Geometry check sheet. Reference: the model listing, model coordinates, mm. A direction names the side the tool comes from. Round coordinates to 2 decimals unless told otherwise and drop trailing zeros. Order: outer loops, then holes, each group sorted by start corner. A loop starts at its lowest first (then second) coordinate and runs counter-clockwise, first axis right, second up. Notation, with made-up numbers: (-5, 0) - (24, 0) arc R7 cw to (24, 10) - close; hole circle Ø2 at (53.5, 59.25). An arc over 180 degrees is marked (long way). Use a Markdown table: item, result. Add a question column.
(1) Access from +Z, -Z, +X, -X, +Y, -Y to the whole of each face (thin tool, end or side, straight path). Record for faces 4 (the face through (0, -22, 8)), 5 (the face through (12.5, -41, 4)).
(2) Gauge pin test, flat ends, axial feed: P1, Ø4, axis at y = -39.5, z = 6, coming from the -X side; P2, Ø2, axis at x = 10.5, z = 2, coming from the +Y side. Record the tip position at first contact, or that the pin passes through.
(3) Thickness scan on line 1 along Y through (x, z) = (0, 3.75); line 2 along Y through (x, z) = (0, 3.5); line 3 along X through (y, z) = (-49.5, 6). Record the ranges inside material, lowest first. Write a range as [from, to].
(4) Section check B-B on x = 0. Record the boundary of the cut face in (y, z), then the cut area to 3 significant figures.
(5) Section check C-C on y = -57.5. Record the boundary of the cut face in (x, z).
(6) Section check A-A on z = 4. Record the boundary of the cut face in (x, y).
(7) Mould release check, pull along Y, two halves, no side actions. Record for faces 1 (the face through (-14.985, 0.66, 3.944)), 2 (the face through (-12.5, -40, 4)), 3 (the face through (0, -65.612, 4)): released by +Y, released by -Y, zero draft, split by the parting line, or undercut.
(8) Section check D-D on x = 4.5. Record the boundary of the cut face in (y, z), then the cut area to 3 significant figures.
```python
from build123d import *

# Parameters (mm, degrees)
F0_R     = 15
F1_DEPTH = 8
F3_D     = 6


with BuildPart() as f1:
    # F0 (on Top) → F1 (new body)
    with BuildSketch(Plane.XY):
        with BuildLine():
            ThreePointArc((12.5, -15.612494996), (18.0277563773, -8.6602540378), (20, 0))
            ThreePointArc((20, 0), (-8.6602540378, 18.0277563773), (-12.5, -15.612494996))
            Line((-12.5, -15.612494996), (12.5, -15.612494996))
        make_face()
        Circle(F0_R, mode=Mode.SUBTRACT)
        with BuildLine():
            Line((12.5, -15.612494996), (-12.5, -15.612494996))
            ThreePointArc((-12.5, -15.612494996), (0, -20), (12.5, -15.612494996))
        make_face()
        with BuildLine():
            ThreePointArc((12.5, -15.612494996), (0, -20), (-12.5, -15.612494996))
            Line((-12.5, -15.612494996), (-12.5, -65.612494996))
            Line((-12.5, -65.612494996), (12.5, -65.612494996))
            Line((12.5, -65.612494996), (12.5, -15.612494996))
        make_face()
    extrude(amount=F1_DEPTH)

    # F3 (through all)
    with Locations(Plane.YZ.offset(12.5)):
        with Locations((-55.612494996, 4)):
            Hole(F3_D / 2)


solid = f1.part
```
Check sheet entries:
| question | item | result |
|---|---|---|
| 1 | face 4 | +Z, +X, -X, +Y, -Y |
| 1 | face 5 | +Z, -Z, +X, -Y |
| 2 | P1 | stops at x = -12.5 |
| 2 | P2 | stops at y = 17.6 |
| 3 | line 1 | y = [-65.61, -58.6], [-52.62, -15], [15, 20] |
| 3 | line 2 | y = [-65.61, -58.57], [-52.65, -15], [15, 20] |
| 3 | line 3 | x = [-12.5, 12.5] |
| 4 | outline | (-65.61, 0) - (-15, 0) - (-15, 8) - (-65.61, 8) - close; (15, 0) - (20, 0) - (20, 8) - (15, 8) - close; hole circle Ø6 at (-55.61, 4) |
| 4 | area | 417 mm2 |
| 5 | outline | (-12.5, 0) - (12.5, 0) - (12.5, 1.67) - (-12.5, 1.67) - close; (-12.5, 6.33) - (12.5, 6.33) - (12.5, 8) - (-12.5, 8) - close |
| 6 | outline | (-12.5, -65.61) - (12.5, -65.61) - (12.5, -58.61) - (-12.5, -58.61) - close; (-12.5, -52.61) - (12.5, -52.61) - (12.5, -15.61) arc R20 ccw (long way) to (-12.5, -15.61) - close; hole circle Ø30 at (0, 0) |
| 7 | face 1 | undercut |
| 7 | face 2 | zero draft |
| 7 | face 3 | released by -Y |
| 8 | outline | (-65.61, 0) - (-14.31, 0) - (-14.31, 8) - (-65.61, 8) - close; (14.31, 0) - (19.49, 0) - (19.49, 8) - (14.31, 8) - close; hole circle Ø6 at (-55.61, 4) |
| 8 | area | 424 mm2 |
